Source: CAD feature listing. Evaluate the final solid. Frame: model axes, mm. A direction names the side the tool comes from. Coordinates: 2 decimals unless noted, no trailing zeros. Order: outer loops, then holes, each group sorted by start corner. A loop starts at its lowest first (then second) coordinate and runs counter-clockwise, first axis right, second up.
```python
from build123d import *

# Parameters (mm, degrees)
BOSS_EXTRUDE1_DEPTH = 1
BOSS_EXTRUDE2_DEPTH = 2.7
SKETCH5_OUTSIDE_W   = 198.872
SKETCH5_OUTSIDE_H   = 130.378
SKETCH5_OUTSIDE_R   = 3
CUT_EXTRUDE1_DEPTH  = 2


with BuildPart() as part:
    # Sketch3 → Boss-Extrude1 (new body)
    with BuildSketch(Plane(origin=(0, 0, 0), x_dir=(1, 0, 0), z_dir=(0, 1, 0))):
        Polygon((-80, 45), (80, 45), (80, -46.505636843), (-80, -45), align=None)
    extrude(amount=BOSS_EXTRUDE1_DEPTH)

    # Sketch4 → Boss-Extrude2 (add)
    with BuildSketch(Plane.XZ):
        with BuildLine():
            Line((-70.35, 37.979513383), (-70.35, 32.020486617))
            add(Edge.make_bspline(
                [(-70.35, 37.979513383), (-73.35, 37.979513383), (-73.35, 35), (-73.35, 32.020486617), (-70.35, 32.020486617)],
                knots=[4.71238898, 4.71238898, 4.71238898, 6.283185307, 6.283185307, 7.853981634, 7.853981634, 7.853981634], degree=2, weights=[1, 0.707106781, 1, 0.707106781, 1]))
        make_face()
        with BuildLine():
            Line((-69.65, 37.979513383), (-69.65, 32.020486617))
            add(Edge.make_bspline(
                [(-69.65, 32.020486617), (-66.65, 32.020486617), (-66.65, 35), (-66.65, 37.979513383), (-69.65, 37.979513383)],
                knots=[4.71238898, 4.71238898, 4.71238898, 6.283185307, 6.283185307, 7.853981634, 7.853981634, 7.853981634], degree=2, weights=[1, 0.707106781, 1, 0.707106781, 1]))
        make_face()
        with BuildLine():
            Line((69.65, 37.979513383), (69.65, 32.020486617))
            add(Edge.make_bspline(
                [(69.65, 37.979513383), (66.65, 37.979513383), (66.65, 35), (66.65, 32.020486617), (69.65, 32.020486617)],
                knots=[4.71238898, 4.71238898, 4.71238898, 6.283185307, 6.283185307, 7.853981634, 7.853981634, 7.853981634], degree=2, weights=[1, 0.707106781, 1, 0.707106781, 1]))
        make_face()
        with BuildLine():
            Line((70.35, 37.979513383), (70.35, 32.020486617))
            add(Edge.make_bspline(
                [(70.35, 32.020486617), (73.35, 32.020486617), (73.35, 35), (73.35, 37.979513383), (70.35, 37.979513383)],
                knots=[4.71238898, 4.71238898, 4.71238898, 6.283185307, 6.283185307, 7.853981634, 7.853981634, 7.853981634], degree=2, weights=[1, 0.707106781, 1, 0.707106781, 1]))
        make_face()
        with BuildLine():
            Line((69.65, -32.020486617), (69.65, -37.979513383))
            add(Edge.make_bspline(
                [(69.65, -32.020486617), (66.65, -32.020486617), (66.65, -35), (66.65, -37.979513383), (69.65, -37.979513383)],
                knots=[4.71238898, 4.71238898, 4.71238898, 6.283185307, 6.283185307, 7.853981634, 7.853981634, 7.853981634], degree=2, weights=[1, 0.707106781, 1, 0.707106781, 1]))
        make_face()
        with BuildLine():
            Line((70.35, -32.020486617), (70.35, -37.979513383))
            add(Edge.make_bspline(
                [(70.35, -37.979513383), (73.35, -37.979513383), (73.35, -35), (73.35, -32.020486617), (70.35, -32.020486617)],
                knots=[4.71238898, 4.71238898, 4.71238898, 6.283185307, 6.283185307, 7.853981634, 7.853981634, 7.853981634], degree=2, weights=[1, 0.707106781, 1, 0.707106781, 1]))
        make_face()
        with BuildLine():
            Line((-70.35, -32.020486617), (-70.35, -37.979513383))
            add(Edge.make_bspline(
                [(-70.35, -32.020486617), (-73.35, -32.020486617), (-73.35, -35), (-73.35, -37.979513383), (-70.35, -37.979513383)],
                knots=[4.71238898, 4.71238898, 4.71238898, 6.283185307, 6.283185307, 7.853981634, 7.853981634, 7.853981634], degree=2, weights=[1, 0.707106781, 1, 0.707106781, 1]))
        make_face()
        with BuildLine():
            Line((-69.65, -32.020486617), (-69.65, -37.979513383))
            add(Edge.make_bspline(
                [(-69.65, -37.979513383), (-66.65, -37.979513383), (-66.65, -35), (-66.65, -32.020486617), (-69.65, -32.020486617)],
                knots=[4.71238898, 4.71238898, 4.71238898, 6.283185307, 6.283185307, 7.853981634, 7.853981634, 7.853981634], degree=2, weights=[1, 0.707106781, 1, 0.707106781, 1]))
        make_face()
    extrude(amount=BOSS_EXTRUDE2_DEPTH)

    # Sketch5 outside → Cut-Extrude1 (cut)
    with BuildSketch(Plane.XZ):
        with Locations((0, 0.753)):
            Rectangle(SKETCH5_OUTSIDE_W, SKETCH5_OUTSIDE_H)
        with Locations((-70, 35)):
            Circle(SKETCH5_OUTSIDE_R, mode=Mode.SUBTRACT)
        with Locations((70, 35)):
            Circle(SKETCH5_OUTSIDE_R, mode=Mode.SUBTRACT)
        with Locations((70, -35)):
            Circle(SKETCH5_OUTSIDE_R, mode=Mode.SUBTRACT)
        with Locations((-70, -35)):
            Circle(SKETCH5_OUTSIDE_R, mode=Mode.SUBTRACT)
    extrude(amount=CUT_EXTRUDE1_DEPTH, mode=Mode.SUBTRACT)


solid = part.part
```
Q1. Section query A-A on y = -0.6. Output: boundary loops of the cut face in (x, z), plus the area to 3 significant figures.
Solutions:
outline: (-70.35, -37.98) - (-70.35, -32.02) arc R3 ccw to start; (-70.35, 32.02) - (-70.35, 37.98) arc R3 ccw to start; (-69.65, -37.98) arc R3 ccw to (-69.65, -32.02) - close; (-69.65, 32.02) arc R3 ccw to (-69.65, 37.98) - close; (69.65, -37.98) - (69.65, -32.02) arc R3 ccw to start; (69.65, 32.02) - (69.65, 37.98) arc R3 ccw to start; (70.35, -37.98) arc R3 ccw to (70.35, -32.02) - close; (70.35, 32.02) arc R3 ccw to (70.35, 37.98) - close
area: 96.3 mm2
Q2. Set-up query: faces 1 (the flat face through (-73.2, -2, -35)), 2 (the flat face through (73.2, -2, -35)), 3 (the flat face through (-66.8, -2, -35)), 4 (the flat face through (-71, -2.7, -35)). Return all of +Z, -Z, +X, -X, +Y, -Y with unobstructed straight access to the full face (end or side cutting, diameter ignored); none if empty.
Solutions:
face 1: -X
face 2: +X
face 3: none
face 4: +Z, -Z, +X, -X, -Y
Q3. Section query C-C on x = -32. Output: boundary loops of the cut face in (y, z), plus the area to 3 significant figures.
Solutions:
outline: (0, -45) - (1, -45) - (1, 45.45) - (0, 45.45) - close
area: 90.5 mm2
Q4. Pull-direction query (Y, two-part tool) for faces 5 (the flat face through (1, 1, 0)), 6 (the flat face through (73.2, -2, 35)), 7 (the flat face through (69, -2.7, -35)); classes: pulls with the +Y half, pulls with the -Y half, needs draft (parallel to the pull), parting line crosses it, or undercut.
Solutions:
face 5: pulls with the +Y half
face 6: undercut
face 7: pulls with the -Y half
Q5. Pin query (flat end, axial travel): P1, Ø8, axis at x = -35.5, z = 26.5, coming from the -Y side; P2, Ø1.4, axis at y = -1.5, z = 34.5, coming from the +X side; P3, Ø0.8, axis at y = -2, z = -36, coming from the -X side. Return the tip coordinate at first contact, or that it passes through.
Solutions:
P1: stops at y = 0
P2: stops at x = 73.35
P3: stops at x = -73.29
Q6. Material intervals for line 1 along Y through (x, z) = (5, 16.5); line 2 along Z through (x, y) = (-69, 0.15); line 3 along Z through (x, y) = (40, 0.75), sorted ascending.
Solutions:
line 1: y = 0 to 1
line 2: z = -45 to 45.1
line 3: z = -45 to 46.13
Q7. Section query B-B on z = 18. Output: boundary loops of the cut face in (x, y), plus the area to 3 significant figures.
Solutions:
outline: (-80, 0) - (80, 0) - (80, 1) - (-80, 1) - close
area: 160 mm2
